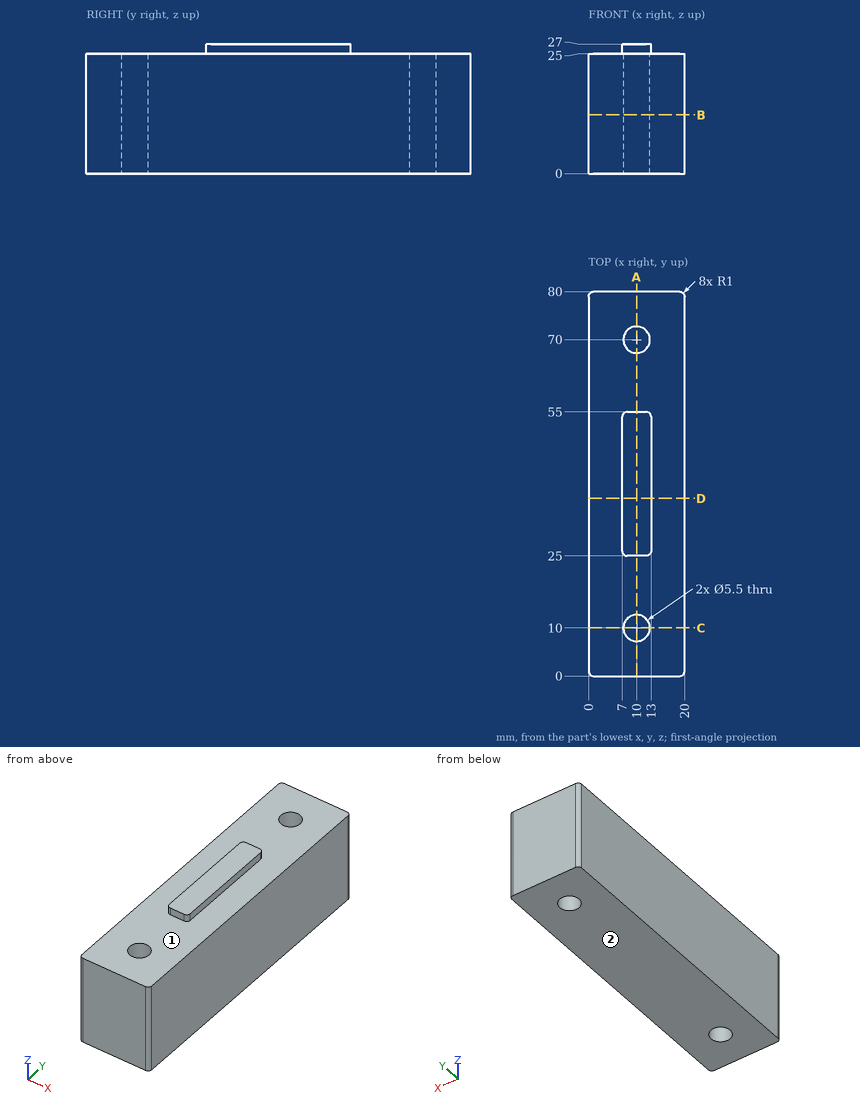
Input: dimensioned drawing with shaded views. Units: mm. Origin: part minimum x, y, z. A direction names the side the tool comes from. Coordinates: 2 decimals unless noted, no trailing zeros. Order: outer loops, then holes, each group sorted by start corner. A loop starts at its lowest first (then second) coordinate and runs counter-clockwise, first axis right, second up.
Item 1: Access query for the marked faces 1 and 2. Directions: +Z, -Z, +X, -X, +Y, -Y. A direction counts if a zero-diameter tool reaches every point of the face in a straight line with its end or side. Return the directions, or none.
Answer:
face 1: +Z
face 2: -Z, +X, -X, +Y, -Y
Item 2: Section query C-C (y = 10). Output: boundary loops of the cut face in (x, z).
Answer:
outline: (0, 0) - (7.25, 0) - (7.25, 25) - (0, 25) - close; (12.75, 0) - (20, 0) - (20, 25) - (12.75, 25) - close
Item 3: Section query A-A (x = 10). Output: boundary loops of the cut face in (y, z), then the cut area to 4 significant figures.
Answer:
outline: (0, 0) - (7.25, 0) - (7.25, 25) - (0, 25) - close; (12.75, 0) - (67.25, 0) - (67.25, 25) - (55, 25) - (55, 27) - (25, 27) - (25, 25) - (12.75, 25) - close; (72.75, 0) - (80, 0) - (80, 25) - (72.75, 25) - close
area: 1,785 mm2
Item 4: Section query D-D (y = 37). Output: boundary loops of the cut face in (x, z).
Answer:
outline: (0, 0) - (20, 0) - (20, 25) - (13, 25) - (13, 27) - (7, 27) - (7, 25) - (0, 25) - close
Item 5: Section query B-B (z = 12.25). Output: boundary loops of the cut face in (x, y), then the cut area to 3 significant figures.
Answer:
outline: (0, 1) arc R1 ccw to (1, 0) - (19, 0) arc R1 ccw to (20, 1) - (20, 79) arc R1 ccw to (19, 80) - (1, 80) arc R1 ccw to (0, 79) - close; hole circle Ø5.5 at (10, 10); hole circle Ø5.5 at (10, 70)
area: 1,550 mm2
Item 6: Contact query for flat-ended pins moving along their axis: P1, Ø1.5, axis at x = 15, y = 13.5, coming from the +Z side; P2, Ø1, axis at x = 9, z = 26, coming from the -Y side; P3, Ø1.6, axis at x = 9.5, z = 26, coming from the +Y side. Output: stop coordinate, or through.
Answer:
P1: stops at z = 25
P2: stops at y = 25
P3: stops at y = 55
Item 7: Material intervals for line 1 along Y through (x, z) = (10, 11.75); line 2 along Z through (x, y) = (6.5, 74); line 3 along X through (y, z) = (68.5, 13.5), sorted ascending.
Answer:
line 1: y = 0 to 7.25, 12.75 to 67.25, 72.75 to 80
line 2: z = 0 to 25
line 3: x = 0 to 7.7, 12.3 to 20
